Design review of the part built by this model. Coordinates are the model's own, in mm. A direction names the side the tool comes from. Give positions to 0.01 mm unless a question says otherwise; leave off trailing zeros. Write each loop counter-clockwise with the first axis right and the second up, starting at its lowest first coordinate (ties: lowest second). Pieces come first, ordered by that corner, then holes. Notation, with made-up numbers: (55, 41.25) -> (63, 41.25) arc R18 ccw to (63, 75.25) -> close; hole circle Ø1 at (69.5, 53.25). An arc over 180 degrees is marked (long way). Answer as a JSON object with one key per item and string values.
```python
from build123d import *

# Parameters (mm, degrees)
SKETCH1_W           = 50
SKETCH1_H           = 200
BOSS_EXTRUDE1_DEPTH = 15
SKETCH2_R           = 5
CUT_EXTRUDE2_DEPTH  = 16
SKETCH3_W           = 50
SKETCH3_H           = 15
BOSS_EXTRUDE2_DEPTH = 50
SKETCH4_W           = 50
SKETCH4_H           = 15
BOSS_EXTRUDE3_DEPTH = 50
SKETCH5_R           = 5
CUT_EXTRUDE3_DEPTH  = 16


with BuildPart() as part:
    # Sketch1 → Boss-Extrude1 (new body)
    with BuildSketch(Plane(origin=(0, 0, 0), x_dir=(1, 0, 0), z_dir=(0, 1, 0))):
        with Locations((25, 100)):
            Rectangle(SKETCH1_W, SKETCH1_H)
    extrude(amount=BOSS_EXTRUDE1_DEPTH)

    # Sketch2 → Cut-Extrude2 (cut, through all)
    with BuildSketch(Plane(origin=(0, 15, 0), x_dir=(1, 0, 0), z_dir=(0, 1, 0))):
        with Locations((25, 180)):
            Circle(SKETCH2_R)
    extrude(amount=-CUT_EXTRUDE2_DEPTH, mode=Mode.SUBTRACT)

    # Sketch3 → Boss-Extrude2 (add)
    with BuildSketch(Plane(origin=(50, 0, 0), x_dir=(0, 0, -1), z_dir=(1, 0, 0))):
        with Locations((25, 7.5)):
            Rectangle(SKETCH3_W, SKETCH3_H)
    extrude(amount=BOSS_EXTRUDE2_DEPTH)

    # Sketch4 → Boss-Extrude3 (add)
    with BuildSketch(Plane.ZY):
        with Locations((-25, 7.5)):
            Rectangle(SKETCH4_W, SKETCH4_H)
    extrude(amount=BOSS_EXTRUDE3_DEPTH)

    # Sketch5 → Cut-Extrude3 (cut, through all)
    with BuildSketch(Plane(origin=(0, 15, 0), x_dir=(1, 0, 0), z_dir=(0, 1, 0))):
        with Locations((25, 25)):
            Circle(SKETCH5_R)
        with Locations((5, 25)):
            Circle(SKETCH5_R)
        with Locations((-15, 25)):
            Circle(SKETCH5_R)
        with Locations((45, 25)):
            Circle(SKETCH5_R)
        with Locations((65, 25)):
            Circle(SKETCH5_R)
    extrude(amount=-CUT_EXTRUDE3_DEPTH, mode=Mode.SUBTRACT)


solid = part.part
```
(1) We need section B-B, the plane z = -25. State the section outline as (x, y) points.
Here are the results:
{"outline": "(-50, 0) -> (-20, 0) -> (-20, 15) -> (-50, 15) -> close; (-10, 0) -> (0, 0) -> (0, 15) -> (-10, 15) -> close; (10, 0) -> (20, 0) -> (20, 15) -> (10, 15) -> close; (30, 0) -> (40, 0) -> (40, 15) -> (30, 15) -> close; (50, 0) -> (60, 0) -> (60, 15) -> (50, 15) -> close; (70, 0) -> (100, 0) -> (100, 15) -> (70, 15) -> close"}
(2) We need section D-D, the plane x = 65. State the section outline as (y, z) points, then the cut area to 3 significant figures.
Here are the results:
{"outline": "(0, -50) -> (15, -50) -> (15, -30) -> (0, -30) -> close; (0, -20) -> (15, -20) -> (15, 0) -> (0, 0) -> close", "area": "600 mm²"}
(3) We need section A-A, the plane x = 5. State the section outline as (y, z) points, then the cut area to 3 significant figures.
Here are the results:
{"outline": "(0, -200) -> (15, -200) -> (15, -30) -> (0, -30) -> close; (0, -20) -> (15, -20) -> (15, 0) -> (0, 0) -> close", "area": "2,850 mm²"}
(4) We need section C-C, the plane y = 7. State the section outline as (x, z) points, then the cut area to 3 significant figures.
Here are the results:
{"outline": "(-50, -50) -> (0, -50) -> (0, -200) -> (50, -200) -> (50, -50) -> (100, -50) -> (100, 0) -> (-50, 0) -> close; hole circle Ø10 at (-15, -25); hole circle Ø10 at (5, -25); hole circle Ø10 at (25, -180); hole circle Ø10 at (25, -25); hole circle Ø10 at (45, -25); hole circle Ø10 at (65, -25)", "area": "14,500 mm²"}
(5) For faces 5 (the flat face through (0, 7, -124)), 6 (the flat face through (75, 7, -50)), 7 (the cylindrical face through (-16.08, 7.6, -20.12)), list the 3-axis set-ups (+Z, -Z, +X, -X, +Y, -Y) from which the entire face can be reached by the end or side of a thin tool; tool diameter is ignored.
Here are the results:
{"face 5": "-Z, -X, +Y, -Y", "face 6": "-Z, +X, +Y, -Y", "face 7": "+Y, -Y"}
(6) For line 1 along X through (y, z) = (8, -25); line 2 along Z through (x, y) = (25, 8); line 3 along Z through (x, y) = (-15, 9.25), list the stretches that pass through material, from the lowest coordinate up.
Here are the results:
{"line 1": "x = -50 to -20, -10 to 0, 10 to 20, 30 to 40, 50 to 60, 70 to 100", "line 2": "z = -200 to -185, -175 to -30, -20 to 0", "line 3": "z = -50 to -30, -20 to 0"}
(7) Clearance check with flat-ended pins moving along their axes: pin 1 (9 mm diameter, centred on x = -15, z = -25, fed in from -Y); pin 2 (5 mm diameter, centred on x = -25.5, y = 11.5, fed in from -Z); pin 3 (4.5 mm diameter, centred on y = 6.5, z = -142.5, fed in from -X); pin 4 (4.5 mm diameter, centred on y = 5, z = -125, fed in from +X). State where each tip first meets the part, or that it passes through.
Here are the results:
{"pin 1": "passes through", "pin 2": "stops at z = -50", "pin 3": "stops at x = 0", "pin 4": "stops at x = 50"}
(8) The part is to be moulded in two halves that separate along X. For faces 1 (the flat face through (26, 15, -79)), 2 (the flat face through (-50, 8, -25)), 3 (the flat face through (100, 8, -25)), 4 (the cylindrical face through (41, 8, -22)), say which applies: +X half, -X half, draft (parallel to the pull), parting line (faces both ways), or undercut.
Here are the results:
{"face 1": "draft", "face 2": "-X half", "face 3": "+X half", "face 4": "undercut"}
